Here's how the part is built. I have some questions about the finished solid (model axes, mm). Round coordinates to 2 decimals unless told otherwise and drop trailing zeros. Loops run counter-clockwise (first coordinate to the right, second up) from the corner with the lowest first, then second, coordinate; pieces in that order, holes last. Notation, with made-up numbers: (25.25, 71) - (79.25, 71) arc R6 cw to (79.25, 77) - close; hole circle Ø6 at (80, 72). An arc over 180 degrees is marked (long way). Answer as a JSON object with one key per item and string values. Group by question number.
1) Will these pins go through, and if not, where does the flat tip stop? P1, Ø1, axis at y = 3.5, z = 59.5, coming from the +X side; P2, Ø1, axis at x = -15, z = 93, coming from the -Y side; P3, Ø2, axis at x = -12.5, z = 37.5, coming from the +Y side; P4, Ø6, axis at x = -37.5, y = -19, coming from the -Z side.
2) I want a section at A-A, the plane z = 23. Please give me the cut outline in (x, y), then the cut area to 3 significant figures.
3) If I drill on line 1 along X through (y, z) = (-1, 18); line 2 along Y through (x, z) = (2, 20); line 3 along Y through (x, z) = (6, 68), over which ranges is the centre line in solid material (lowest first)? Write a range as [from, to].
4) I want a section at B-B, the plane x = 15. Please give me the cut outline in (y, z).
5) I want a section at C-C, the plane y = -33. Please give me the cut outline in (x, z), then the cut area to 3 significant figures.
from build123d import *

# Parameters (mm, degrees)
F0_R     = 53.5223969486
F1_DEPTH = 113.03
F2_DEPTH = 42.418
F3_R     = 36.0053843075
F4_DEPTH = 25.4
F5_DEPTH = 25.4


with BuildPart() as f1:
    # F0 (on Top) → F1 (new body)
    with BuildSketch(Plane.XY):
        Circle(F0_R)
    extrude(amount=F1_DEPTH)

    # F2 (add): a face of the model
    f2_faces = [f1.faces().sort_by_distance(p)[0] for p in [
        (0, 0, 113.03),
    ]]
    extrude(f2_faces, amount=F2_DEPTH)

    # F3 (on face) → F4 (join)
    with BuildSketch(Plane.XY.offset(155.448)):
        Circle(F3_R)
    extrude(amount=F4_DEPTH)

    # F5 (add): a face of the model
    f5_faces = [f1.faces().sort_by_distance(p)[0] for p in [
        (-52.0085549555, 0, 155.448),
    ]]
    extrude(f5_faces, amount=F5_DEPTH)


solid = f1.part
Outcome:
{
 "1": {"P1": "x = 53.44", "P2": "y = -51.52", "P3": "y = 52.27", "P4": "z = 0"},
 "2": {"outline": "circle Ø107.04 at (0, 0)", "area": "9,000 mm^2"},
 "3": {"line 1": "[-53.51, 53.51]", "line 2": "[-53.49, 53.49]", "line 3": "[-53.19, 53.19]"},
 "4": {"outline": "(-51.38, 0) - (51.38, 0) - (51.38, 180.85) - (-51.38, 180.85) - close"},
 "5": {"outline": "(-42.14, 0) - (42.14, 0) - (42.14, 180.85) - (-42.14, 180.85) - close", "area": "15,200 mm^2"}
}
